Geometry: final body of the model. Coordinates: model frame, mm. Face numbers are marked on the shaded views. A direction names the side the tool comes from. Give positions to 0.01 mm unless a question says otherwise; leave off trailing zeros. Write each loop counter-clockwise with the first axis right and the second up, starting at its lowest first coordinate (ties: lowest second). Pieces come first, ordered by that corner, then holes.
Q1. Line query: L1, parallel to Y at x = 5.5, z = 3.75; L2, parallel to X at y = -20.5, z = 5.25; L3, parallel to X at y = -10, z = 9 (3 decimals). Output: solid intervals per line, ascending.
Q2. Cut plane D-D on z = 8.25. Count the separate pieces of the cut face and the enclosed holes in it, plus the area to 3 significant figures.
Q3. Cut plane C-C on x = -27. Return the cut outline in (y, z), plus the area to 3 significant figures.
Q4. Draft query along Y for the marked faces 1, 2, 3 and 4. Return one class per face: pulls with the +Y half, pulls with the -Y half, needs draft (parallel to the pull), parting line crosses it, or undercut.
Q5. Cut plane A-A on x = -2. Return the cut outline in (y, z).
Q6. Cut plane B-B on y = -27.5. Return the cut outline in (x, z), plus the area to 3 significant figures.
Q7. Pin query (flat end, axial travel): pin 1 (1 mm diameter, centred on x = 22, z = 8.5, fed in from -Y); pin 2 (6 mm diameter, centred on x = -19, z = 3.5, fed in from -Y); pin 3 (5 mm diameter, centred on x = -38, z = 8.5, fed in from -Y). Return the tip coordinate at first contact, or that it passes through.
Q8. Reachability of the marked faces 5, 6 and 7 from +Z, -Z, +X, -X, +Y, -Y: full face, straight path, thin tool, end or side. Return the list, or none.
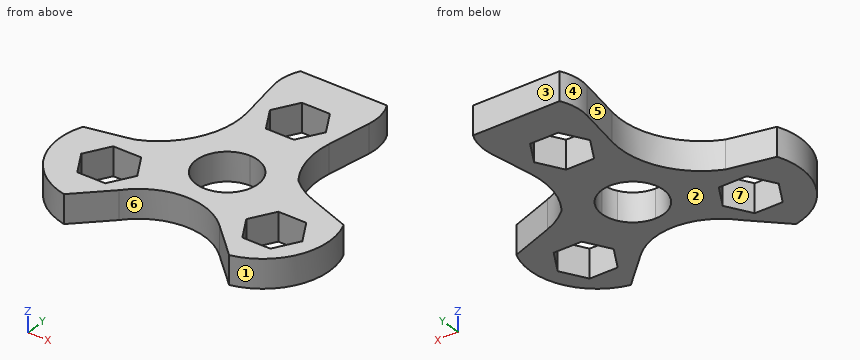
```python
from build123d import *

# Parameters (mm, degrees)
F1_DEPTH = 10.16
F2_DEPTH = 10.16


with BuildPart() as f1:
    # F0 (on Top) → F1 (new body)
    with BuildSketch(Plane.XY):
        with BuildLine():
            Line((-31.7672, -1.802307), (-47.777991, -5.121411))
            Line((-47.777991, -5.121411), (-30.534543, -37.468957))
            Line((-30.534543, -37.468957), (-19.185807, -26.351705))
            ThreePointArc((-19.185807, -26.351705), (-2.4424, -17.805796), (15.218731, -24.244639))
            Line((15.218731, -24.244639), (27.066497, -35.513725))
            ThreePointArc((27.066497, -35.513725), (43.090442, -23.144741), (43.831861, -2.915829))
            Line((43.831861, -2.915829), (28.491493, 2.762567))
            ThreePointArc((28.491493, 2.762567), (23.536918, 5.15939), (19.131085, 8.458057))
            ThreePointArc((19.131085, 8.458057), (14.766541, 18.537353), (14.508489, 29.518011))
            Line((14.508489, 29.518011), (17.181797, 45.178168))
            ThreePointArc((17.181797, 45.178168), (17.224125, 50.784528), (15.484437, 56.114307))
            Line((15.484437, 56.114307), (-15.484437, 56.114307))
            ThreePointArc((-15.484437, 56.114307), (-17.224125, 50.784528), (-17.181797, 45.178168))
            Line((-17.181797, 45.178168), (-14.508489, 29.518011))
            ThreePointArc((-14.508489, 29.518011), (-17.662338, 10.840635), (-31.7672, -1.802307))
        make_face()
        Polygon((-24.499209, -8.366125), (-21.997045, -12.7), (-19.494881, -17.033875), (-24.499209, -25.701625), (-34.507865, -25.701625), (-39.512193, -17.033875), (-34.507865, -8.366125), align=None, mode=Mode.SUBTRACT)
        Polygon((19.496714, -17.0307), (21.997045, -12.7), (24.497376, -8.3693), (24.499209, -8.366125), (34.507865, -8.366125), (39.512193, -17.033875), (34.507865, -25.701625), (24.499209, -25.701625), (19.494881, -17.033875), align=None, mode=Mode.SUBTRACT)
        with BuildLine():
            ThreePointArc((-9.524721, -5.4991), (-9.524721, 5.4991), (0, 10.9982))
            ThreePointArc((0, 10.9982), (7.776902, 7.776902), (10.9982, 0))
            ThreePointArc((10.9982, 0), (10.623445, -2.846544), (9.524721, -5.4991))
            ThreePointArc((9.524721, -5.4991), (5.4991, -9.524721), (0, -10.9982))
            ThreePointArc((0, -10.9982), (-5.4991, -9.524721), (-9.524721, -5.4991))
        make_face(mode=Mode.SUBTRACT)
        Polygon((5.004328, 25.4), (0, 25.4), (-5.004328, 25.4), (-10.008656, 34.06775), (-5.004328, 42.7355), (5.004328, 42.7355), (10.008656, 34.06775), align=None, mode=Mode.SUBTRACT)
    extrude(amount=F1_DEPTH)

    # F0 (on Top) → F2 (join)
    with BuildSketch(Plane.XY):
        with BuildLine():
            Line((-30.534543, -37.468957), (-47.777991, -5.121411))
            ThreePointArc((-47.777991, -5.121411), (-46.738845, -25.337215), (-30.534543, -37.468957))
        make_face()
    extrude(amount=F2_DEPTH)


solid = f1.part
```
Data:
1. L1: y = -18.68 to -9.52, 9.52 to 26.26, 41.88 to 56.11
1. L2: x = -48.67 to -37.51, -21.5 to -12.02, 10.01 to 21.5, 37.51 to 44.25
1. L3: x = -49.183 to -35.451, -23.556 to -4.578, 4.578 to 23.556, 35.451 to 45.625
2. separate pieces: 1
2. enclosed holes: 4
2. area: 3,230 mm2
3. outline: (-34.01, 0) - (-25.7, 0) - (-25.7, 10.16) - (-34.01, 10.16) - close; (-8.37, 0) - (0.73, 0) - (0.73, 10.16) - (-8.37, 10.16) - close
3. area: 177 mm2
4. face 1: parting line crosses it
4. face 2: needs draft
4. face 3: pulls with the +Y half
4. face 4: undercut
5. outline: (-17.78, 0) - (-10.81, 0) - (-10.81, 10.16) - (-17.78, 10.16) - close; (10.81, 0) - (25.4, 0) - (25.4, 10.16) - (10.81, 10.16) - close; (42.74, 0) - (56.11, 0) - (56.11, 10.16) - (42.74, 10.16) - close
6. outline: (-45.43, 0) - (-20.36, 0) - (-20.36, 10.16) - (-45.43, 10.16) - close; (18.64, 0) - (40.21, 0) - (40.21, 10.16) - (18.64, 10.16) - close
6. area: 474 mm2
7. pin 1: stops at y = -31.17
7. pin 2: stops at y = -29.11
7. pin 3: stops at y = -35.86
8. face 5: +Z, -Z, -X
8. face 6: +Z, -Z, -Y
8. face 7: +Z, -Z
